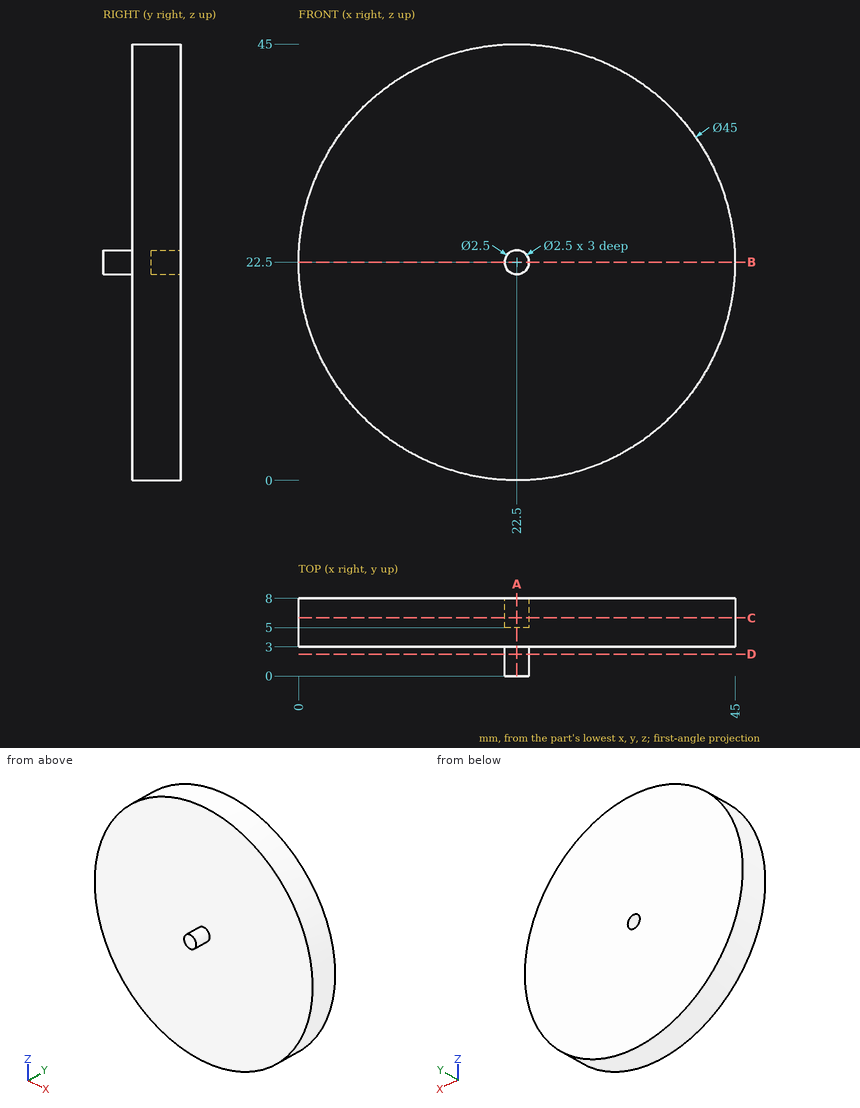
The figure shows three views and two pictorial views of one solid part (mm, origin at its lowest corner). Answer the questions. Coordinates: 2 decimals unless noted, no trailing zeros. Write each loop counter-clockwise with the first axis right and the second up, starting at its lowest first coordinate (ties: lowest second). Pieces come first, ordered by that corner, then holes. Notation, with made-up numbers: (22, 79) -> (33, 79) arc R15 ccw to (33, 100) -> close; hole circle Ø9 at (21, -22). An arc over 180 degrees is marked (long way). Answer as a JSON object with one key per item and string values.
Q1. The part is cut by section A-A on x = 22.5. Give the vertices of the cut face in (y, z), then the cut area to 3 significant figures.
The answers:
{"outline": "(0, 21.25) -> (3, 21.25) -> (3, 0) -> (8, 0) -> (8, 21.25) -> (5, 21.25) -> (5, 23.75) -> (8, 23.75) -> (8, 45) -> (3, 45) -> (3, 23.75) -> (0, 23.75) -> close", "area": "225 mm2"}
Q2. The part is cut by section B-B on z = 22.5. Give the vertices of the cut face in (x, y).
The answers:
{"outline": "(0, 3) -> (21.25, 3) -> (21.25, 0) -> (23.75, 0) -> (23.75, 3) -> (45, 3) -> (45, 8) -> (23.75, 8) -> (23.75, 5) -> (21.25, 5) -> (21.25, 8) -> (0, 8) -> close"}
Q3. The part is cut by section D-D on y = 2.25. Give the vertices of the cut face in (x, z), then the cut area to 3 significant figures.
The answers:
{"outline": "circle Ø2.5 at (22.5, 22.5)", "area": "4.91 mm2"}
Q4. The part is cut by section C-C on y = 6. Give the vertices of the cut face in (x, z), then the cut area to 3 significant figures.
The answers:
{"outline": "circle Ø45 at (22.5, 22.5); hole circle Ø2.5 at (22.5, 22.5)", "area": "1,590 mm2"}
Q5. Flat-ended cylindrical pins translate along their axes: pin 1 Ø1 at (y, z) = (6.5, 27.5) entering from -X; pin 2 Ø1.5 at (x, z) = (38.5, 30) entering from -Y; pin 3 Ø4 at (y, z) = (2, 15) entering from +X. Find the tip coordinate at first contact, or state that the pin passes through.
The answers:
{"pin 1": "stops at x = 0.45", "pin 2": "stops at y = 3", "pin 3": "stops at x = 44.25"}
Q6. Consider line 1 (X direction, y = 6.8, z = 22.5); line 2 (Y direction, x = 4, z = 20). Determine where each line is inside the solid, lowest interval first. Write a range as [from, to].
The answers:
{"line 1": "x = [0, 21.25], [23.75, 45]", "line 2": "y = [3, 8]"}
